Here's the drawing with two shaded views (mm, measured from the low corner). I have some questions. Give positions to 0.01 mm unless a question says otherwise; leave off trailing zeros. Write each loop counter-clockwise with the first axis right and the second up, starting at its lowest first coordinate (ties: lowest second). Pieces come first, ordered by that corner, then holes. Notation, with made-up numbers: (-23, 81.5) - (24, 81.5) arc R9 ccw to (24, 95.5) - close; hole circle Ø9 at (15.25, 15). An arc over 180 degrees is marked (long way). Use one line per item in the form item = value.
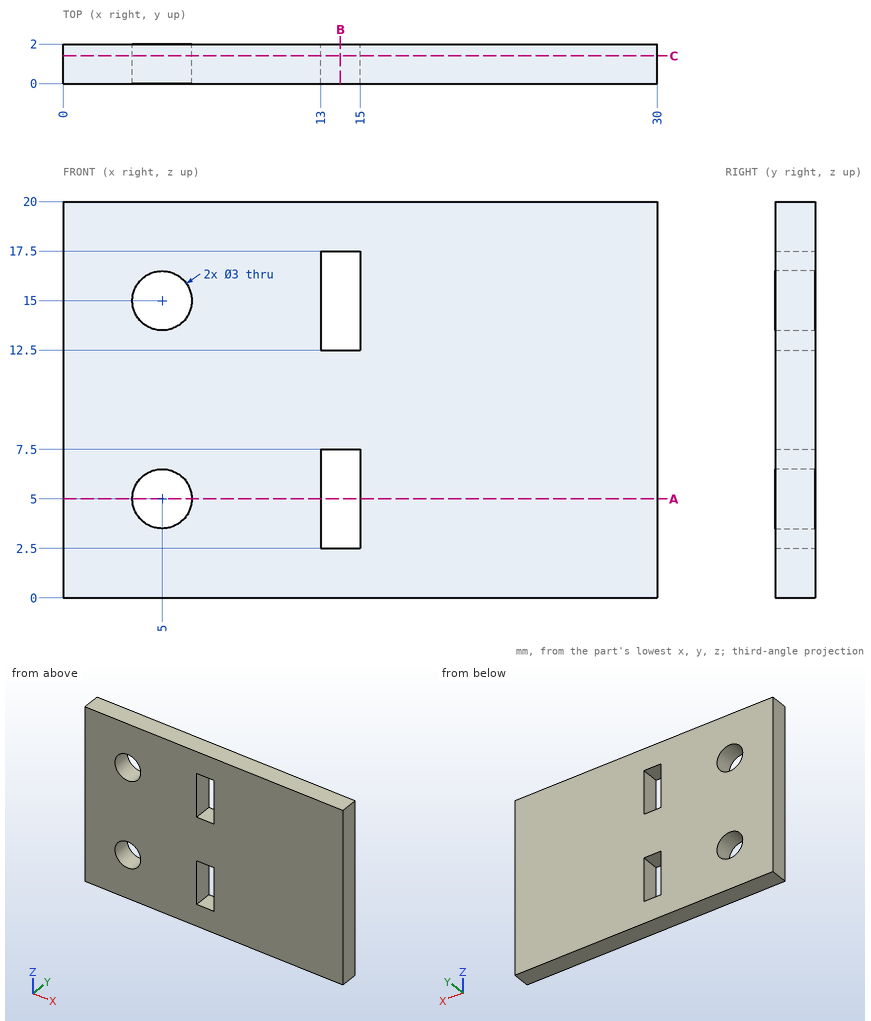
1. Imagine slicing it at B-B, the plane x = 14. List the corners of the cut face in (y, z) for me, and give its area (3 significant figures).
Response values:
outline = (0, 0) - (2, 0) - (2, 2.5) - (0, 2.5) - close; (0, 7.5) - (2, 7.5) - (2, 12.5) - (0, 12.5) - close; (0, 17.5) - (2, 17.5) - (2, 20) - (0, 20) - close
area = 20.0 mm²
2. For pin 1 (1 mm diameter, centred on y = 1, z = 14, fed in from -X), with a flat end and sliding along its axis, tell me the tip position at first contact or that it passes through.
Response values:
pin_1 = 0
3. If I drill on line 1 (X direction, y = 0.8, z = 15); line 2 (Z direction, x = 13.75, y = 0.3); line 3 (X direction, y = 0.25, z = 16), over which ranges is the centre line in solid material (lowest first)? Write a range as from..to.
Response values:
line_1 = 0..3.5, 6.5..13, 15..30
line_2 = 0..2.5, 7.5..12.5, 17.5..20
line_3 = 0..3.88, 6.12..13, 15..30
4. Imagine slicing it at C-C, the plane y = 1.4. List the corners of the cut face in (x, z) for me.
Response values:
outline = (0, 0) - (30, 0) - (30, 20) - (0, 20) - close; hole circle Ø3 at (5, 5); hole circle Ø3 at (5, 15); hole (13, 2.5) - (15, 2.5) - (15, 7.5) - (13, 7.5) - close; hole (13, 12.5) - (15, 12.5) - (15, 17.5) - (13, 17.5) - close
5. Imagine slicing it at A-A, the plane z = 5. List the corners of the cut face in (x, y) for me.
Response values:
outline = (0, 0) - (3.5, 0) - (3.5, 2) - (0, 2) - close; (6.5, 0) - (13, 0) - (13, 2) - (6.5, 2) - close; (15, 0) - (30, 0) - (30, 2) - (15, 2) - close
